Can you work these out from the model? Positions are in its coordinate system, mm. Give positions to 0.01 mm unless a question says otherwise; leave off trailing zeros. Order: outer loops, then holes, each group sorted by start corner. A loop starts at its lowest first (then second) coordinate and runs counter-clockwise, first axis right, second up. Notation, with made-up numbers: M 76.25,-40 L 91.25,-40 A28 ccw 91.25,-17 Z; hole C -15,77 d5. An arc over 180 degrees is marked long. Use one line per item in the form item = value. Start each with the question number.
1. I want a section at C-C, the plane y = -1.2. List the corners of the cut face in (x, z) for me.
2. I want a section at D-D, the plane z = -12. List the corners of the cut face in (x, y) for me.
3. I want a section at A-A, the plane x = -1. List the corners of the cut face in (y, z) for me, and give its area (3 significant figures).
4. I need wall thicknesses on L1, parallel to Z at x = -1, y = -1.25; L2, parallel to Z at x = 2, y = -1.6; L3, parallel to X at y = -0.8, z = -13. Which ranges of each line are inside material? Lowest first, please.
5. I want a section at B-B, the plane z = 11.5. List the corners of the cut face in (x, y) for me, and give its area (3 significant figures).
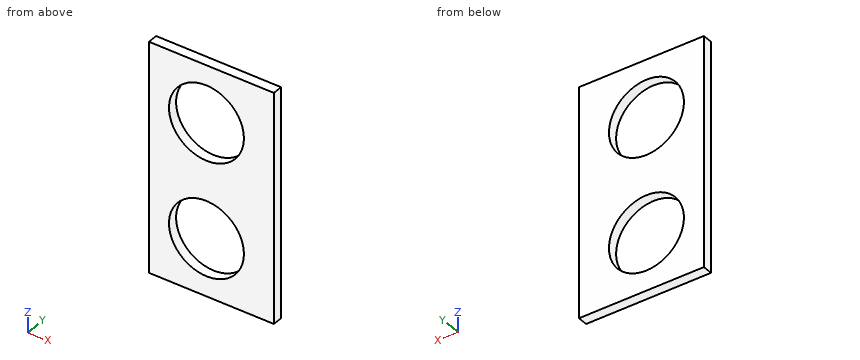
```python
from build123d import *

# Parameters (mm, degrees)
SKETCH_W     = 25
SKETCH_H     = 46
PAD_DEPTH    = 2
SKETCH001_R  = 7.5
POCKET_DEPTH = 5


with BuildPart() as part:
    # Sketch → Pad (new body)
    with BuildSketch(Plane.XZ):
        Rectangle(SKETCH_W, SKETCH_H)
    extrude(amount=PAD_DEPTH)

    # Sketch001 (on Face6 of Pad) → Pocket (cut)
    with BuildSketch(Plane.XZ.offset(2)):
        with Locations((-1, 11.5)):
            Circle(SKETCH001_R)
        with Locations((-1, -11.5)):
            Circle(SKETCH001_R)
    extrude(amount=-POCKET_DEPTH, mode=Mode.SUBTRACT)


solid = part.part
```
Check result:
q1.outline = M -12.5,-23 L 12.5,-23 L 12.5,23 L -12.5,23 Z; hole C -1,-11.5 d15; hole C -1,11.5 d15
q2.outline = M -12.5,-2 L -8.48,-2 L -8.48,0 L -12.5,0 Z; M 6.48,-2 L 12.5,-2 L 12.5,0 L 6.48,0 Z
q3.outline = M -2,-23 L 0,-23 L 0,-19 L -2,-19 Z; M -2,-4 L 0,-4 L 0,4 L -2,4 Z; M -2,19 L 0,19 L 0,23 L -2,23 Z
q3.area = 32.0 mm2
q4.L1 = -23 to -19, -4 to 4, 19 to 23
q4.L2 = -23 to -18.37, -4.63 to 4.63, 18.37 to 23
q4.L3 = -12.5 to -8.35, 6.35 to 12.5
q5.outline = M -12.5,-2 L -8.5,-2 L -8.5,0 L -12.5,0 Z; M 6.5,-2 L 12.5,-2 L 12.5,0 L 6.5,0 Z
q5.area = 20.0 mm2
